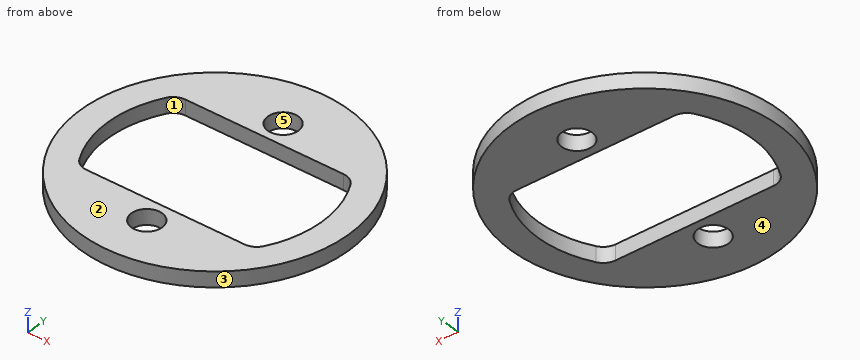
```python
from build123d import *

# Parameters (mm, degrees)
SKETCH1_R           = 17.5
SKETCH1_R_2         = 13.97
SKETCH1_R_3         = 2
BOSS_EXTRUDE1_DEPTH = 2
FILLET1_R           = 2


with BuildPart() as part:
    # Sketch1 → Boss-Extrude1 (new body)
    # profile 1 of 3: a face of its own
    with BuildSketch(Plane.XY):
        Circle(SKETCH1_R)
        Circle(SKETCH1_R_2, mode=Mode.SUBTRACT)
    # profile 2 of 3: a face of its own
    with BuildSketch(Plane.XY):
        with BuildLine():
            Line((11.473447607, -7.97), (-11.473447607, -7.97))
            ThreePointArc((-11.473447607, -7.97), (0, -13.97), (11.473447607, -7.97))
        make_face()
        with Locations((0, -10.97)):
            Circle(SKETCH1_R_3, mode=Mode.SUBTRACT)
    # profile 3 of 3: a face of its own
    with BuildSketch(Plane.XY):
        with BuildLine():
            Line((-11.473447607, 7.97), (11.473447607, 7.97))
            ThreePointArc((11.473447607, 7.97), (0, 13.97), (-11.473447607, 7.97))
        make_face()
        with Locations((0, 10.97)):
            Circle(SKETCH1_R_3, mode=Mode.SUBTRACT)
    extrude(amount=BOSS_EXTRUDE1_DEPTH)

    # Fillet1
    fillet1_edges = [part.edges().sort_by_distance(p)[0] for p in [
        (11.473447607, -7.97, 1),
        (11.473447607, 7.97, 1),
        (-11.473447607, 7.97, 1),
        (-11.473447607, -7.97, 1),
    ]]
    fillet(fillet1_edges, radius=FILLET1_R)


solid = part.part
```
Can you work these out from the model? Positions are in its coordinate system, mm. Face numbers are marked on the shaded views. A direction names the side the tool comes from. Coordinates: 2 decimals unless noted, no trailing zeros. Loops run counter-clockwise (first coordinate to the right, second up) from the corner with the lowest first, then second, coordinate; pieces in that order, holes last. Notation, with made-up numbers: (-7.5, 32.25) -> (12.5, 32.25) arc R38 cw to (12.5, 71.25) -> close; hole circle Ø10 at (21, 8). An arc over 180 degrees is marked (long way). Answer as a JSON object with one key per item and string values.
1) For the marked faces 1 and 2, which set-ups out of +Z, -Z, +X, -X, +Y, -Y let a thin tool reach every point of the face, with its end or its side?
Results:
{"face 1": "+Z, -Z", "face 2": "+Z, +X, -X, +Y, -Y"}
2) Imagine slicing it at A-A (x = 5.5). Please give me the cut outline in (y, z).
Results:
{"outline": "(-16.61, 0) -> (-7.97, 0) -> (-7.97, 2) -> (-16.61, 2) -> close; (7.97, 0) -> (16.61, 0) -> (16.61, 2) -> (7.97, 2) -> close"}
3) Imagine slicing it at D-D (x = 0). Please give me the cut outline in (y, z).
Results:
{"outline": "(-17.5, 0) -> (-12.97, 0) -> (-12.97, 2) -> (-17.5, 2) -> close; (-8.97, 0) -> (-7.97, 0) -> (-7.97, 2) -> (-8.97, 2) -> close; (7.97, 0) -> (8.97, 0) -> (8.97, 2) -> (7.97, 2) -> close; (12.97, 0) -> (17.5, 0) -> (17.5, 2) -> (12.97, 2) -> close"}
4) For P1, Ø5, axis at x = 0, y = 10.97, coming from the +Z side; P2, Ø0.6, axis at x = -2.5, z = 0.5, coming from the -Y side; P3, Ø1, axis at x = -13.5, z = 1.5, coming from the -Y side; P4, Ø0.6, axis at x = -1, z = 1, coming from the +Y side, each with a flat end and sliding along its axis, tell me the tip position at first contact or that it passes through.
Results:
{"P1": "stops at z = 2", "P2": "stops at y = -17.36", "P3": "stops at y = -11.72", "P4": "stops at y = 17.49"}
5) Imagine slicing it at C-C (z = 1.2). Please give me the cut outline in (x, y).
Results:
{"outline": "circle Ø35 at (0, 0); hole (-12.11, -6.97) arc R2 ccw to (-10.37, -7.97) -> (10.37, -7.97) arc R2 ccw to (12.11, -6.97) arc R13.97 ccw to (12.11, 6.97) arc R2 ccw to (10.37, 7.97) -> (-10.37, 7.97) arc R2 ccw to (-12.11, 6.97) arc R13.97 ccw to start; hole circle Ø4 at (0, -10.97); hole circle Ø4 at (0, 10.97)"}
6) Imagine slicing it at B-B (y = -12.5). Please give me the cut outline in (x, z), then the cut area to 3 significant figures.
Results:
{"outline": "(-12.25, 0) -> (-1.29, 0) -> (-1.29, 2) -> (-12.25, 2) -> close; (1.29, 0) -> (12.25, 0) -> (12.25, 2) -> (1.29, 2) -> close", "area": "43.8 mm^2"}
7) If I drill on line 1 (Y direction, x = 0, z = 0.5); line 2 (X direction, y = 0.5, z = 0.7); line 3 (Y direction, x = -8, z = 0.4), over which ranges is the centre line in solid material (lowest first)?
Results:
{"line 1": "y = -17.5 to -12.97, -8.97 to -7.97, 7.97 to 8.97, 12.97 to 17.5", "line 2": "x = -17.49 to -13.96, 13.96 to 17.49", "line 3": "y = -15.56 to -7.97, 7.97 to 15.56"}
8) Thinking about a two-plate mould opening in Y: for the marked faces 3, 4 and 5, which applies, pulls with the +Y half, pulls with the -Y half, needs draft (parallel to the pull), parting line crosses it, or undercut?
Results:
{"face 3": "parting line crosses it", "face 4": "needs draft", "face 5": "undercut"}
